The drawing under review shows one solid part. Ordinate dimensions are in mm from its lowest x, y, z. A direction names the side the tool comes from. Coordinates: 2 decimals unless noted, no trailing zeros. Write each loop counter-clockwise with the first axis right and the second up, starting at its lowest first coordinate (ties: lowest second). Pieces come first, ordered by that corner, then holes. Notation, with made-up numbers: (23.5, 2.25) - (52.5, 2.25) arc R15 ccw to (52.5, 8.25) - close; hole circle Ø6 at (-15.5, 36.25). An arc over 180 degrees is marked (long way). Use a Markdown table: item, result.
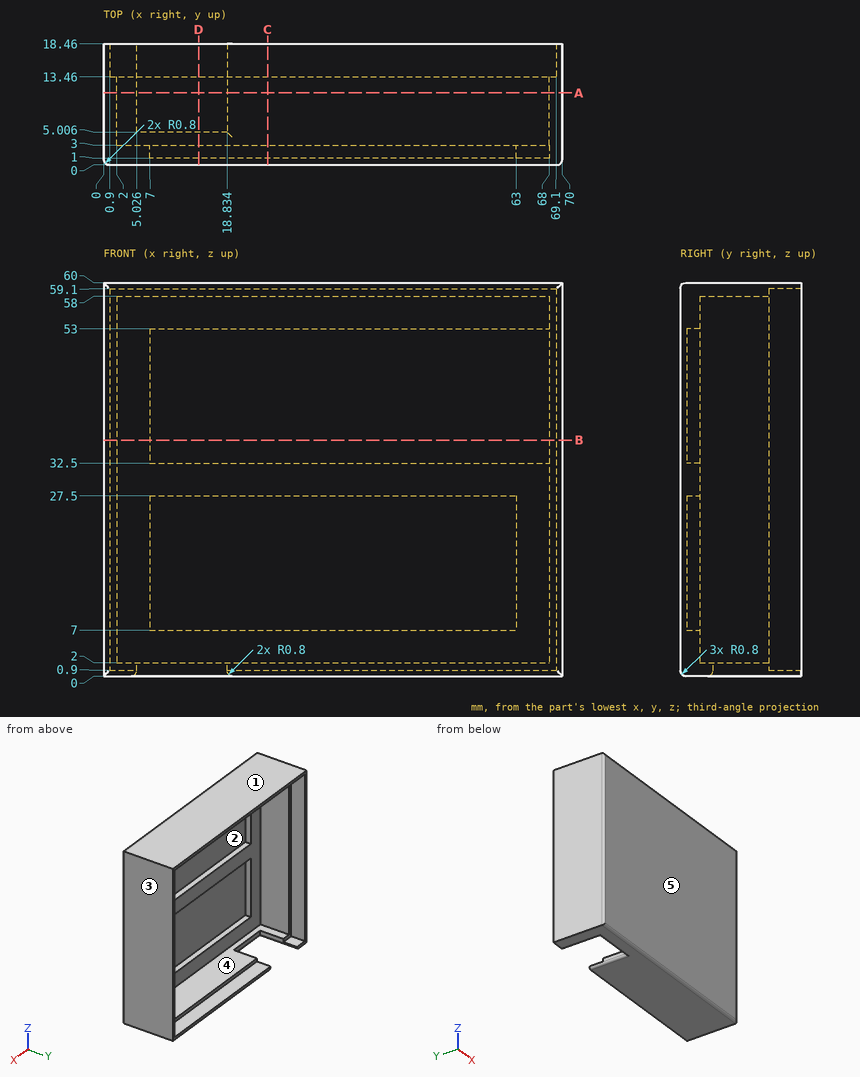
(1) For L1, parallel to Z at x = 60, y = 2.75; L2, parallel to X at y = 6.25, z = 18; L3, parallel to Z at x = 43, y = 12, list the stretches that pass through material, from the lowest coordinate up. Write a range as from..to.
Determined:
| item | result |
|---|---|
| L1 | 0..7, 27.5..32.5, 53..60 |
| L2 | 0..2, 68..70 |
| L3 | 0..2, 58..60 |
(2) Take a section at D-D on x = 14.5. Write out the cut boundary in (y, z), and give its area (3 significant figures).
Determined:
| item | result |
|---|---|
| outline | (0, 0.8) arc R0.8 ccw to (0.8, 0) - (4.21, 0) arc R0.8 ccw to (5.01, 0.8) - (5.01, 2) - (3, 2) - (3, 7) - (1, 7) - (1, 27.5) - (3, 27.5) - (3, 32.5) - (1, 32.5) - (1, 53) - (3, 53) - (3, 58) - (13.46, 58) - (13.46, 59.1) - (18.46, 59.1) - (18.46, 60) - (0.8, 60) arc R0.8 ccw to (0, 59.2) - close |
| area | 127 mm2 |
(3) Take a section at C-C on x = 25. Write out the cut boundary in (y, z).
Determined:
| item | result |
|---|---|
| outline | (0, 0.8) arc R0.8 ccw to (0.8, 0) - (18.46, 0) - (18.46, 0.9) - (13.46, 0.9) - (13.46, 2) - (3, 2) - (3, 7) - (1, 7) - (1, 27.5) - (3, 27.5) - (3, 32.5) - (1, 32.5) - (1, 53) - (3, 53) - (3, 58) - (13.46, 58) - (13.46, 59.1) - (18.46, 59.1) - (18.46, 60) - (0.8, 60) arc R0.8 ccw to (0, 59.2) - close |
(4) For pin 1 (1.5 mm diameter, centred on x = 17, z = 8.5, fed in from +Y); pin 2 (0.6 mm diameter, centred on x = 9, z = 1.5, fed in from +Y); pin 3 (10 mm diameter, centred on x = 43.5, z = 24.5, fed in from +Y), all flat-tipped, find the tip position at first contact; note any pin that passes through.
Determined:
| item | result |
|---|---|
| pin 1 | y = 1 |
| pin 2 | y = 5.01 |
| pin 3 | y = 3 |
(5) Draft analysis for pull direction X (two halves, no side actions). For the marked faces 3, 4 and 5, state which applies: +X half, -X half, draft (parallel to the pull), parting line (faces both ways), or undercut.
Determined:
| item | result |
|---|---|
| face 3 | +X half |
| face 4 | undercut |
| face 5 | draft |
(6) Take a section at A-A on y = 11. Write out the cut boundary in (x, z).
Determined:
| item | result |
|---|---|
| outline | (0, 0) - (4.23, 0) arc R0.8 ccw to (5.03, 0.8) - (5.03, 2) - (2, 2) - (2, 58) - (68, 58) - (68, 2) - (18.83, 2) - (18.83, 0.8) arc R0.8 ccw to (19.63, 0) - (70, 0) - (70, 60) - (0, 60) - close |
(7) Machinability: for the marked faces 1 and 2, which of the approach directions +Z, -Z, +X, -X, +Y, -Y give a long, thin tool a straight path to every point of the face, cutting with its end or side? Answer none if there is none.
Determined:
| item | result |
|---|---|
| face 1 | +Z, +X, -X, +Y, -Y |
| face 2 | +Y |
(8) Take a section at B-B on z = 36. Write out the cut boundary in (x, y).
Determined:
| item | result |
|---|---|
| outline | (0, 0.8) arc R0.8 ccw to (0.8, 0) - (69.2, 0) arc R0.8 ccw to (70, 0.8) - (70, 18.46) - (69.1, 18.46) - (69.1, 13.46) - (68, 13.46) - (68, 1) - (7, 1) - (7, 3) - (2, 3) - (2, 13.46) - (0.9, 13.46) - (0.9, 18.46) - (0, 18.46) - close |
